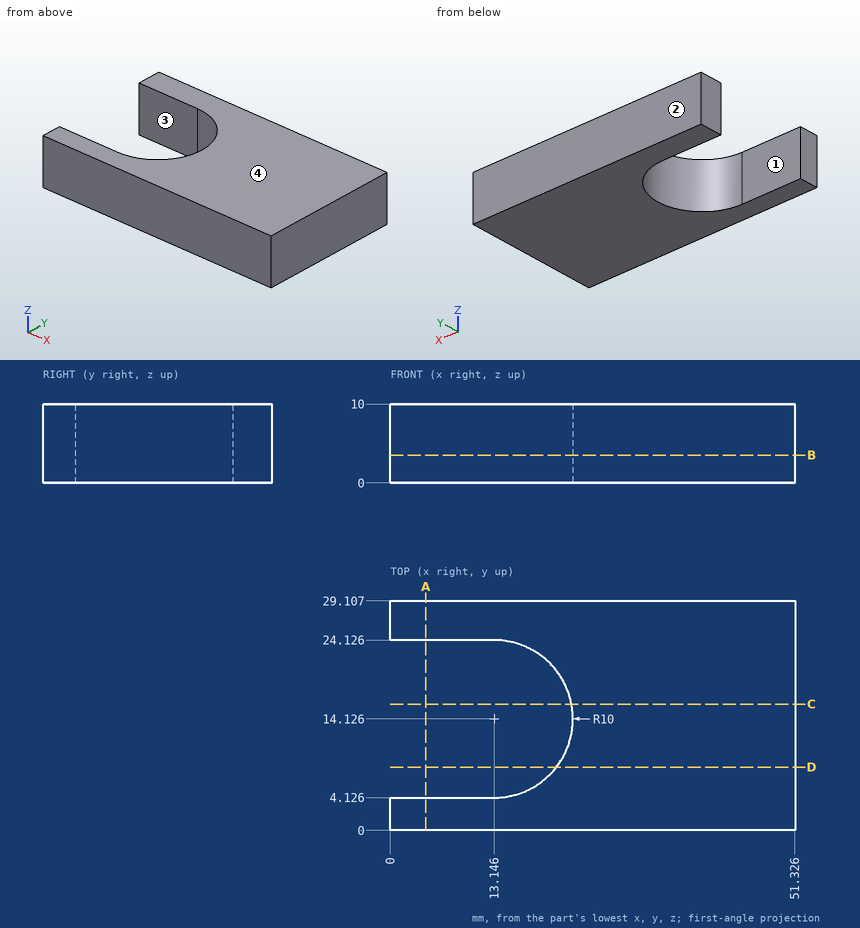
Here's the drawing with two shaded views (mm, measured from the low corner). I have some questions. Coordinates: 2 decimals unless noted, no trailing zeros. Order: outer loops, then holes, each group sorted by start corner. A loop starts at its lowest first (then second) coordinate and runs counter-clockwise, first axis right, second up. Notation, with made-up numbers: (-3.75, 32.25) - (23.25, 32.25) arc R10 ccw to (23.25, 49.25) - close; hole circle Ø3 at (-1, 13.25). An arc over 180 degrees is marked (long way). Answer in a Markdown table with one row per item. Add a question column.
(1) If we mould it in two halves opening along Y, with no side actions, what happens to the marked faces 1, 2, 3 and 4? For each: released by +Y, released by -Y, zero draft, split by the parting line, or undercut.
(2) If we section it at D-D, the plane y = 8: Please give me the cut outline in (x, z), then the cut area to 3 significant figures.
(3) If we section it at B-B, the plane z = 3.5: Please give me the cut outline in (x, y).
(4) If we section it at C-C, the plane y = 16: Please give me the cut outline in (x, z), then the cut area to 3 significant figures.
(5) I need wall thicknesses on L1, parallel to Y at x = 8, z = 5; L2, parallel to X at y = 14, z = 8.25 (1 decimal); L3, parallel to Y at x = 14.5, z = 5.5 (1 decimal). Which ranges of each line are inside material? Lowest first, please.
(6) If we section it at A-A, the plane x = 4.5: Please give me the cut outline in (y, z).
(7) Will this pin go through, and if not, where does the flat tip stop? pin 1 (10 mm diameter, centred on x = 13, y = 16, fed in from +Z).
Results are:
| question | item | result |
|---|---|---|
| 1 | face 1 | undercut |
| 1 | face 2 | released by +Y |
| 1 | face 3 | undercut |
| 1 | face 4 | zero draft |
| 2 | outline | (21.05, 0) - (51.33, 0) - (51.33, 10) - (21.05, 10) - close |
| 2 | area | 303 mm2 |
| 3 | outline | (0, 0) - (51.33, 0) - (51.33, 29.11) - (0, 29.11) - (0, 24.13) - (13.15, 24.13) arc R10 cw to (13.15, 4.13) - (0, 4.13) - close |
| 4 | outline | (22.97, 0) - (51.33, 0) - (51.33, 10) - (22.97, 10) - close |
| 4 | area | 284 mm2 |
| 5 | L1 | y = 0 to 4.13, 24.13 to 29.11 |
| 5 | L2 | x = 23.1 to 51.3 |
| 5 | L3 | y = 0 to 4.2, 24 to 29.1 |
| 6 | outline | (0, 0) - (4.13, 0) - (4.13, 10) - (0, 10) - close; (24.13, 0) - (29.11, 0) - (29.11, 10) - (24.13, 10) - close |
| 7 | pin 1 | passes through |
